from build123d import *

# Parameters (mm, degrees)
F1_DEPTH = 6
F2_R     = 10
F3_DEPTH = 30.67
F4_DEPTH = 30.8
F5_DEPTH = 29.7
F6_W     = 30
F6_H     = 11
F6_W_2   = 30.67
F6_H_2   = 9
F7_DEPTH = 6
F8_R     = 1.5
F9_DEPTH = 37.3


with BuildPart() as f1:
    # F0 (on Top) → F1 (new body)
    with BuildSketch(Plane.XY):
        Polygon((120, 17.5), (-150, 17.5), (-150, -17.5), (120, -17.5), (120, -8.5), (0, -8.5), (0, -6.5), (150, -6.5), (150, 4.5), (0, 4.5), (0, 6.5), (120, 6.5), align=None)
    extrude(amount=F1_DEPTH)

    # F2
    f2_edges = [f1.edges().sort_by_distance(p)[0] for p in [
        (-150, -17.5, 3),
        (-150, 17.5, 3),
    ]]
    fillet(f2_edges, radius=F2_R)

    # F3 (add): a face of the model
    f3_faces = [f1.faces().sort_by_distance(p)[0] for p in [
        (120, -13, 3),
    ]]
    extrude(f3_faces, amount=F3_DEPTH)

    # F4 (add): a face of the model
    f4_faces = [f1.faces().sort_by_distance(p)[0] for p in [
        (120, 12, 3),
    ]]
    extrude(f4_faces, amount=F4_DEPTH)

    # F5 (cut): a face of the model
    f5_faces = [f1.faces().sort_by_distance(p)[0] for p in [
        (150, -1, 3),
    ]]
    extrude(f5_faces, amount=-F5_DEPTH, mode=Mode.SUBTRACT)

    # F6 (on face) → F7 (join)
    with BuildSketch(Plane.XY.offset(6)):
        with Locations((135.8, 12)):
            Rectangle(F6_W, F6_H)
        with Locations((135.335, -13)):
            Rectangle(F6_W_2, F6_H_2)
    extrude(amount=F7_DEPTH)

    # F8 (on face) → F9 (cut)
    with BuildSketch(Plane.XZ.offset(17.5)):
        with Locations((140.17, 6)):
            Circle(F8_R)
    extrude(amount=-F9_DEPTH, mode=Mode.SUBTRACT)


solid = f1.part
Input: part model. Units: mm. Frame: model coordinates. A direction names the side the tool comes from. Round coordinates to 2 decimals unless told otherwise and drop trailing zeros. Loops run counter-clockwise (first coordinate to the right, second up) from the corner with the lowest first, then second, coordinate; pieces in that order, holes last. Notation, with made-up numbers: (6.25, -21) -> (39.25, -21) arc R28 ccw to (39.25, 17) -> close; hole circle Ø6 at (-40, 78). An arc over 180 degrees is marked (long way). Answer as a JSON object with one key per item and string values. Group by question number.
1) Section query B-B on y = -12.5. Output: boundary loops of the cut face in (x, z).
2) Reachability of faces 1 (the cylindrical face through (-147.15, -14.49, 3.04)), 2 (the flat face through (120.3, -1, 3)), 3 (the flat face through (120, -13, 9)), 4 (the flat face through (120.8, 12, 9)) from +Z, -Z, +X, -X, +Y, -Y: full face, straight path, thin tool, end or side. Return the list, or none.
3) Section query C-C on x = -114. Output: boundary loops of the cut face in (y, z), plus the area to 3 significant figures.
4) Section query A-A on x = 36.5. Output: boundary loops of the cut face in (y, z).
5) Pin query (flat end, axial travel): pin 1 (1.8 mm diameter, centred on x = 140.17, z = 6, fed in from -Y); pin 2 (1.5 mm diameter, centred on y = 11, z = 4, fed in from -X); pin 3 (3 mm diameter, centred on y = -11.5, z = 10.5, fed in from +X); pin 4 (0.6 mm diameter, centred on y = 5.5, z = 4, fed in from +X). Return the tip coordinate at first contact, or that it passes through.
6) Ray query, L1, parallel to Y at x = 92, z = 1; L2, parallel to Z at x = 140.17, y = -12.5; L3, parallel to X at y = 8, z = 5.75. Return the intervals inside material, ascending.
7) Draft query along Y for faces 5 (the cylindrical face through (-146.99, 14.65, 3.04)), 6 (the flat face through (-16, 0, 6)), 7 (the flat face through (61, 4.5, 3)), 8 (the flat face through (59, -6.5, 3)). Return one class per face: +Y half, -Y half, draft (parallel to the pull), parting line (faces both ways), or undercut.
Reply:
{
 "1": {"outline": "(-148.66, 0) -> (150.67, 0) -> (150.67, 12) -> (120, 12) -> (120, 6) -> (-148.66, 6) -> close; hole circle Ø3 at (140.17, 6)"},
 "2": {"face 1": "+Z, -Z, -X, -Y", "face 2": "+Z, -Z, +X", "face 3": "+Z, -X, +Y, -Y", "face 4": "+Z, -X, +Y"},
 "3": {"outline": "(-17.5, 0) -> (17.5, 0) -> (17.5, 6) -> (-17.5, 6) -> close", "area": "210 mm2"},
 "4": {"outline": "(-17.5, 0) -> (-8.5, 0) -> (-8.5, 6) -> (-17.5, 6) -> close; (-6.5, 0) -> (4.5, 0) -> (4.5, 6) -> (-6.5, 6) -> close; (6.5, 0) -> (17.5, 0) -> (17.5, 6) -> (6.5, 6) -> close"},
 "5": {"pin 1": "passes through", "pin 2": "stops at x = -149.61", "pin 3": "stops at x = 150.67", "pin 4": "stops at x = 0"},
 "6": {"L1": "y = -17.5 to -8.5, -6.5 to 4.5, 6.5 to 17.5", "L2": "z = 0 to 4.5, 7.5 to 12", "L3": "x = -149.99 to 138.69, 141.65 to 150.8"},
 "7": {"face 5": "+Y half", "face 6": "draft", "face 7": "undercut", "face 8": "undercut"}
}
